```python
from build123d import *

# Parameters (mm, degrees)
ESQUISSE1_R        = 13
ESQUISSE1_R_2      = 1.75
BOSS_EXTRU_1_DEPTH = 11


with BuildPart() as part:
    # Esquisse1 → Boss.-Extru.1 (new body)
    with BuildSketch(Plane.XY):
        Polygon((0, 25), (0, 6), (-8, 6), (-8, 0), (0, 0), (0, -5), (34, -5), (34, 0), (42, 0), (42, 6), (34, 6), (34, 25), (34, 34), (42, 34), (42, 40), (34, 40), (34, 45), (0, 45), (0, 40), (-8, 40), (-8, 34), (0, 34), align=None)
        with Locations((17, 13.5)):
            Circle(ESQUISSE1_R, mode=Mode.SUBTRACT)
        with Locations((3, 23)):
            Circle(ESQUISSE1_R_2, mode=Mode.SUBTRACT)
        with Locations((31, 23)):
            Circle(ESQUISSE1_R_2, mode=Mode.SUBTRACT)
        with Locations((31, 4)):
            Circle(ESQUISSE1_R_2, mode=Mode.SUBTRACT)
        with Locations((3, 4)):
            Circle(ESQUISSE1_R_2, mode=Mode.SUBTRACT)
    extrude(amount=BOSS_EXTRU_1_DEPTH)


solid = part.part
```
Build history of the part. All positions in model axes, mm. A direction names the side the tool comes from. Give positions to 0.01 mm unless a question says otherwise; leave off trailing zeros. Order: outer loops, then holes, each group sorted by start corner. A loop starts at its lowest first (then second) coordinate and runs counter-clockwise, first axis right, second up. Notation, with made-up numbers: M 77.25,40.25 L 95.25,40.25 A30 cw 95.25,71.25 Z; hole C 31.25,18.25 d10. An arc over 180 degrees is marked long. Return JSON: item names as keys, results as strings.
Q1. Two-plate mould, pull along X, no slides. Class faces 4 (the face through (29.71, 24.18, 5.42)), 5 (the face through (42, 37, 5)), 6 (the face through (38, 34, 5)): pulls with the +X half, pulls with the -X half, needs draft (parallel to the pull), parting line crosses it, or undercut.
Answer list:
{"face 4": "undercut", "face 5": "pulls with the +X half", "face 6": "needs draft"}
Q2. Band-saw the part on A-A (x = -1.5). Give the cut face in (y, z).
Answer list:
{"outline": "M 0,0 L 6,0 L 6,11 L 0,11 Z; M 34,0 L 40,0 L 40,11 L 34,11 Z"}
Q3. 3-axis set-ups, long thin cutter, end or side, ignore diameter. For faces 1 (the face through (-4, 34, 5)), 2 (the face through (38, 40, 5)), 3 (the face through (0, 43, 5)): which of +Z, -Z, +X, -X, +Y, -Y reach the whole face in a straight line?
Answer list:
{"face 1": "+Z, -Z, -X", "face 2": "+Z, -Z, +X, +Y", "face 3": "+Z, -Z, -X, +Y"}
Q4. Band-saw the part on C-C (z = 3.75). Give the cut face in (x, y).
Answer list:
{"outline": "M -8,0 L 0,0 L 0,-5 L 34,-5 L 34,0 L 42,0 L 42,6 L 34,6 L 34,34 L 42,34 L 42,40 L 34,40 L 34,45 L 0,45 L 0,40 L -8,40 L -8,34 L 0,34 L 0,6 L -8,6 Z; hole C 3,4 d3.5; hole C 3,23 d3.5; hole C 17,13.5 d26; hole C 31,4 d3.5; hole C 31,23 d3.5"}
Q5. Wall check: probe 1 along Y at (x, z) = (3, 7.5); probe 2 along X at (y, z) = (14, 7); probe 3 along Y at (x, z) = (35.5, 8.25). Give the ranges that are in metal, low to high. Write a range as from..to.
Answer list:
{"probe 1": "y = -5..2.25, 5.75..21.25, 24.75..45", "probe 2": "x = 0..4.01, 29.99..34", "probe 3": "y = 0..6, 34..40"}
Q6. Band-saw the part on B-B (y = 8.5). Give the cut face in (x, z), then the cut area to 3 significant figures.
Answer list:
{"outline": "M 0,0 L 5,0 L 5,11 L 0,11 Z; M 29,0 L 34,0 L 34,11 L 29,11 Z", "area": "110 mm^2"}
Q7. Band-saw the part on D-D (x = 31). Give the cut face in (y, z).
Answer list:
{"outline": "M -5,0 L 2.25,0 L 2.25,11 L -5,11 Z; M 5.75,0 L 21.25,0 L 21.25,11 L 5.75,11 Z; M 24.75,0 L 45,0 L 45,11 L 24.75,11 Z"}
Q8. Flat gauge pins, fed straight in: pin 1 (5.5 mm diameter, centred on x = 3, y = 23, fed in from -Z); pin 2 (2.5 mm diameter, centred on x = -3.5, z = 6.5, fed in from -Y); pin 3 (3.5 mm diameter, centred on y = 26.5, z = 6, fed in from +X); pin 4 (2.5 mm diameter, centred on x = 36.5, z = 5, fed in from +Y). Where does each tip first touch, or does it go through?
Answer list:
{"pin 1": "stops at z = 0", "pin 2": "stops at y = 0", "pin 3": "stops at x = 34", "pin 4": "stops at y = 40"}
